Input: part model. Units: mm. Frame: model coordinates. Round coordinates to 2 decimals unless told otherwise and drop trailing zeros. Loops run counter-clockwise (first coordinate to the right, second up) from the corner with the lowest first, then second, coordinate; pieces in that order, holes last. Notation, with made-up numbers: (47.5, 89.5) - (89.5, 89.5) arc R16 ccw to (89.5, 106.5) - close; hole circle Ø7 at (75, 65.5). An arc over 180 degrees is marked (long way). One line per question, with ' | ' between items. Start each with the question number.
Item 1: Section A-A, the plane y = 3. Return loops of the section in (x, z).
Item 2: First-contact query: pin 1 (2 mm diameter, centred on y = -1, z = -1.5, fed in from -X). Flat tip, straight axial feed; report the tip coordinate or a pass-through.
Item 3: Material intervals for line 1 along Y through (x, z) = (-2, 0.8); line 2 along Y through (x, z) = (-1.6, -1.65); line 3 along Z through (x, y) = (-0.1, -9), sorted ascending.
```python
from build123d import *
from OCP.BRepFilletAPI import BRepFilletAPI_MakeChamfer

# Parameters (mm, degrees)
SKETCH_1_R          = 2.5
EXTRUDE_2_DEPTH     = 22.5
SKETCH_2_R          = 2.5
SKETCH_2_R_2        = 2
CUT_EXTRUDE_1_DEPTH = 0.8
CHAMFER_3_SIZE      = 0.5
CHAMFER_3_SIZE2     = 0.866025404


with BuildPart() as part:
    # 草图1 → 凸台-拉伸2 (new body)
    with BuildSketch(Plane(origin=(0, 0, 0), x_dir=(1, 0, 0), z_dir=(0, 1, 0))):
        with Locations(Location((0, 0, 0), (0, 0, 90))):
            Circle(SKETCH_1_R)
    extrude_2 = extrude(amount=EXTRUDE_2_DEPTH)

    # 草图2 → 切除-拉伸1 (cut)
    with BuildSketch(Plane(origin=(0, 20, 0), x_dir=(1, 0, 0), z_dir=(0, 1, 0))):
        with Locations(Location((0, 0, 0), (0, 0, 90))):
            Circle(SKETCH_2_R)
        with Locations(Location((0, 0, 0), (0, 0, 270))):
            Circle(SKETCH_2_R_2, mode=Mode.SUBTRACT)
    cut_extrude_1 = extrude(amount=CUT_EXTRUDE_1_DEPTH, mode=Mode.SUBTRACT)

    # 镜向3: 凸台-拉伸2 across plane
    add(extrude_2.mirror(Plane.ZX))

    # 镜向5: 切除-拉伸1 across plane
    add(cut_extrude_1.mirror(Plane.ZX), mode=Mode.SUBTRACT)

    # 倒角3: one chamfer whose edges measure the first distance from different faces: ONE call of the kernel's chamfer builder (chamfer() names one face for all edges)
    chamfer_3_edges_1 = [part.edges().sort_by_distance(p)[0] for p in [
        (0, -22.5, 2.5),
    ]]
    chamfer_3_side_1 = [part.faces().sort_by_distance(p)[0] for p in [
        (0, -22.5, 0),
    ]]
    chamfer_3_edges_2 = [part.edges().sort_by_distance(p)[0] for p in [
        (0, 22.5, 2.5),
    ]]
    chamfer_3_side_2 = [part.faces().sort_by_distance(p)[0] for p in [
        (0, 21.65, 2.5),
    ]]
    chamfer_3 = BRepFilletAPI_MakeChamfer(part.part.solid().wrapped)
    for e in chamfer_3_edges_1:
        chamfer_3.Add(CHAMFER_3_SIZE, CHAMFER_3_SIZE2, e.wrapped, chamfer_3_side_1[0].wrapped)  # the first distance lies on this face
    for e in chamfer_3_edges_2:
        chamfer_3.Add(CHAMFER_3_SIZE, CHAMFER_3_SIZE2, e.wrapped, chamfer_3_side_2[0].wrapped)  # the first distance lies on this face
    add(Compound.cast(chamfer_3.Shape()), mode=Mode.REPLACE)


solid = part.part
```
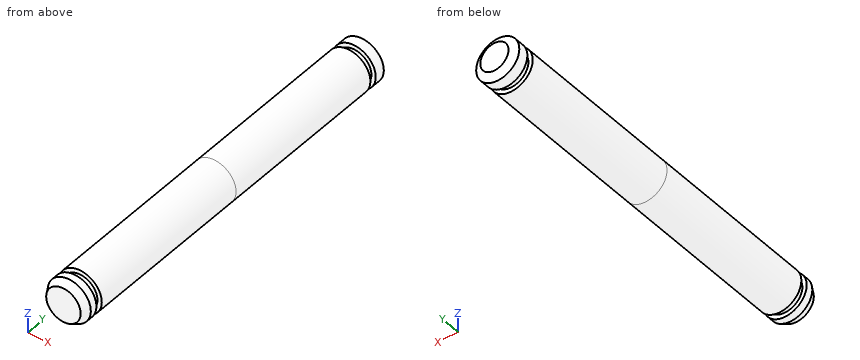
Return value:
1) outline: circle Ø5 at (0, 0)
2) pin 1: x = -2.45
3) line 1: -22.23 to -20.8, -20 to 20, 20.8 to 22.2 | line 2: -21.98 to -20.8, -20 to 20, 20.8 to 22.12 | line 3: -2.5 to 2.5
